```python
from build123d import *

# Parameters (mm, degrees)
SKETCH1_R           = 32.5
BOSS_EXTRUDE1_DEPTH = 20
SKETCH2_R           = 5
CUT_EXTRUDE1_DEPTH  = 1
SKETCH4_R           = 3.05
CUT_EXTRUDE2_DEPTH  = 4.5
SKETCH3_R           = 1.5
CUT_EXTRUDE3_DEPTH  = 2
CUT_EXTRUDE4_START  = -2
SKETCH5_R           = 5
CUT_EXTRUDE4_DEPTH  = 2


with BuildPart() as part:
    # Sketch1 → Boss-Extrude1 (new body)
    with BuildSketch(Plane.XY):
        Circle(SKETCH1_R)
    extrude(amount=BOSS_EXTRUDE1_DEPTH)

    # Sketch2 → Cut-Extrude1 (cut)
    with BuildSketch(Plane.XY.offset(20)):
        Circle(SKETCH2_R)
    extrude(amount=-CUT_EXTRUDE1_DEPTH, mode=Mode.SUBTRACT)

    # Sketch4 → Cut-Extrude2 (cut)
    with BuildSketch(Plane(origin=(0, 0, 0), x_dir=(-1, 0, 0), z_dir=(0, 0, -1))):
        Circle(SKETCH4_R)
    extrude(amount=-CUT_EXTRUDE2_DEPTH, mode=Mode.SUBTRACT)

    # Sketch3 → Cut-Extrude3 (cut)
    with BuildSketch(Plane(origin=(0, 0, 0), x_dir=(-1, 0, 0), z_dir=(0, 0, -1))):
        with Locations((5.5, 9)):
            Circle(SKETCH3_R)
        with Locations((-5.5, 9)):
            Circle(SKETCH3_R)
        with Locations((5.5, -9)):
            Circle(SKETCH3_R)
        with Locations((-5.5, -9)):
            Circle(SKETCH3_R)
    extrude(amount=-CUT_EXTRUDE3_DEPTH, mode=Mode.SUBTRACT)

    # Sketch5 → Cut-Extrude4 (cut)
    with BuildSketch(Plane(origin=(0, 0, 0), x_dir=(-1, 0, 0), z_dir=(0, 0, -1)).offset(CUT_EXTRUDE4_START)):
        with Locations(Location((0, 0, 0), (0, 0, 180))):
            Circle(SKETCH5_R)
    extrude(amount=CUT_EXTRUDE4_DEPTH, mode=Mode.SUBTRACT)


solid = part.part
```
Source: CAD feature listing. Evaluate the final solid. Frame: model axes, mm. A direction names the side the tool comes from. Round coordinates to 2 decimals unless told otherwise and drop trailing zeros. Loops run counter-clockwise (first coordinate to the right, second up) from the corner with the lowest first, then second, coordinate; pieces in that order, holes last. Notation, with made-up numbers: M 82,13.5 L 118,13.5 A24 cw 118,36.5 Z; hole C 70.25,58.25 d8. An arc over 180 degrees is marked long. Put each result on its own line as item: value.
(1) Section B-B, the plane z = 14.25. Return loops of the section in (x, y), and give its area (3 significant figures).
Solutions:
outline: C 0,0 d65
area: 3,320 mm²
(2) Pull-direction query (X, two-part tool) for faces 4 (the face through (7, 0, 0)), 5 (the face through (6, 9, 2)), 6 (the face through (31, 9.76, 9.86)); classes: released by +X, released by -X, zero draft, split by the parting line, or undercut.
Solutions:
face 4: zero draft
face 5: undercut
face 6: split by the parting line
(3) Ray query, line 1 (Y direction, x = 0, z = 19.45); line 2 (Y direction, x = 5.5, z = 1.05); line 3 (Y direction, x = -19.5, z = 10.5). Return the intervals inside material, ascending. Write a range as [from, to].
Solutions:
line 1: [-32.5, -5], [5, 32.5]
line 2: [-32.03, -10.5], [-7.5, 7.5], [10.5, 32.03]
line 3: [-26, 26]
(4) Section C-C, the plane x = 13. Return loops of the section in (y, z), and give its area (3 significant figures).
Solutions:
outline: M -29.79,0 L 29.79,0 L 29.79,20 L -29.79,20 Z
area: 1,190 mm²
(5) Section D-D, the plane y = 9. Return loops of the section in (x, z).
Solutions:
outline: M -31.23,0 L -7,0 L -7,2 L -4,2 L -4,0 L 4,0 L 4,2 L 7,2 L 7,0 L 31.23,0 L 31.23,20 L -31.23,20 Z
(6) First-contact query: pin 1 (8 mm diameter, centred on x = -1.5, y = 1.5, fed in from -Z); pin 2 (2 mm diameter, centred on y = -21.5, z = 2.5, fed in from +X); pin 3 (10 mm diameter, centred on y = 25, z = 11.5, fed in from -X); pin 4 (2.5 mm diameter, centred on x = 5.5, y = -9, fed in from -Z). Flat tips, straight axial feed; report the tip coordinate or a pass-through.
Solutions:
pin 1: z = 0
pin 2: x = 25.22
pin 3: x = -25.62
pin 4: z = 2
(7) Access query for faces 1 (the face through (7, 0, 20)), 2 (the face through (0, 0, 19)), 3 (the face through (-5, 9, 2)). Directions: +Z, -Z, +X, -X, +Y, -Y. A direction counts if a zero-diameter tool reaches every point of the face in a straight line with its end or side. Return the directions, or none.
Solutions:
face 1: +Z, +X, -X, +Y, -Y
face 2: +Z
face 3: -Z
(8) Section A-A, the plane y = 0. Return loops of the section in (x, z).
Solutions:
outline: M -32.5,0 L -5,0 L -5,2 L -3.05,2 L -3.05,4.5 L 3.05,4.5 L 3.05,2 L 5,2 L 5,0 L 32.5,0 L 32.5,20 L 5,20 L 5,19 L -5,19 L -5,20 L -32.5,20 Z
